Could you check a few things on this drawing? It's one solid part, dimensions in mm from its lowest x, y, z. A direction names the side the tool comes from. Coordinates: 2 decimals unless noted, no trailing zeros. Loops run counter-clockwise (first coordinate to the right, second up) from the corner with the lowest first, then second, coordinate; pieces in that order, holes last. Notation, with made-up numbers: (41.25, 17.5) -> (56.25, 17.5) arc R25 ccw to (56.25, 48.5) -> close; hole circle Ø6 at (-26.5, 41). An arc over 180 degrees is marked (long way). One line per question, with ' | ' between items.
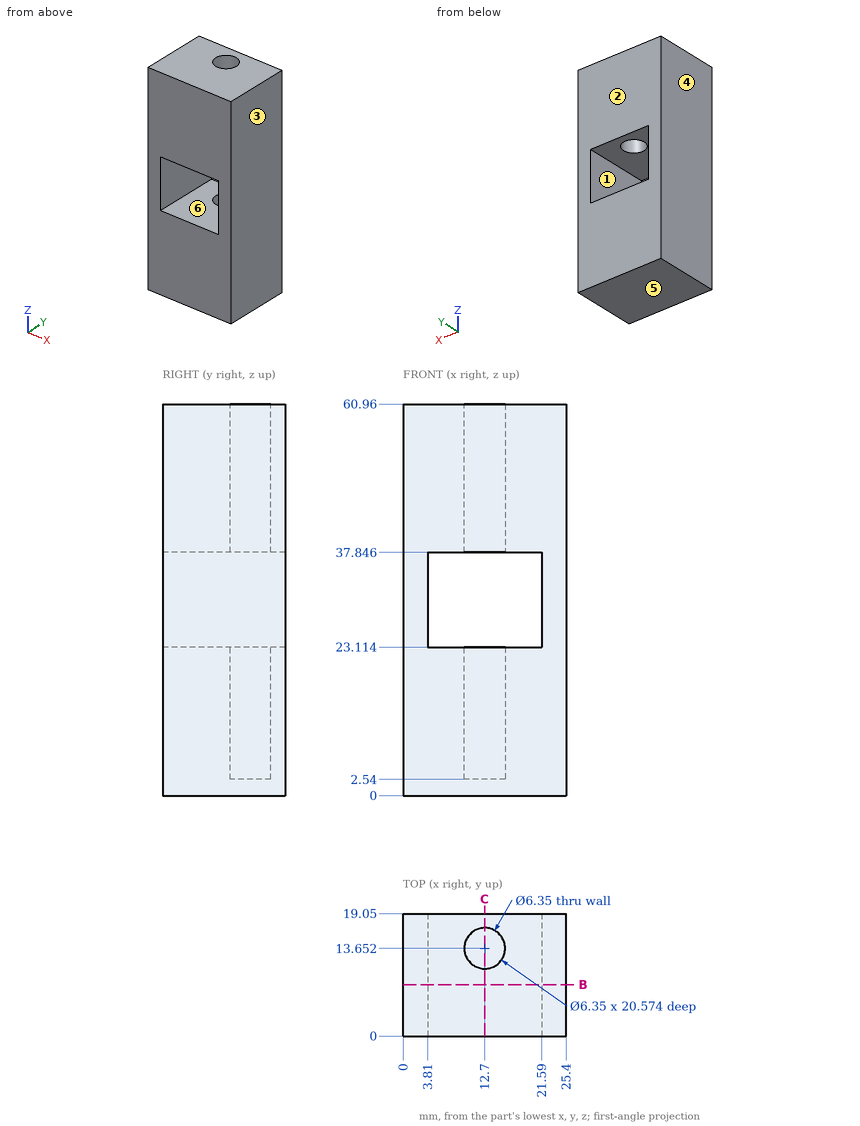
1) If we section it at C-C on x = 12.7: Give the number of separate pieces and of enclosed holes in the cut face, and give its area (3 significant figures).
Data:
separate pieces: 3 | enclosed holes: 0 | area: 603 mm²
2) If we section it at B-B on y = 8: Please give me the cut outline in (x, z) (1 decimal), and give its area (3 significant figures).
Data:
outline: (0, 0) -> (25.4, 0) -> (25.4, 61) -> (0, 61) -> close; hole (3.8, 23.1) -> (21.6, 23.1) -> (21.6, 37.8) -> (3.8, 37.8) -> close | area: 1,290 mm²
3) I need wall thicknesses on line 1 along X through (y, z) = (8.75, 35); line 2 along Z through (x, y) = (5.5, 14.25) (1 decimal); line 3 along Y through (x, z) = (12.7, 48). Which ranges of each line are inside material? Lowest first, please. Write a range as from..to.
Data:
line 1: 0..3.81, 21.59..25.4 | line 2: 0..23.1, 37.8..61 | line 3: 0..10.48, 16.83..19.05
4) On a 3-axis mill with a long thin cutter (end or side, diameter ignored), from which of +Z, -Z, +X, -X, +Y, -Y can I reach the whole of each face in a straight line? I mean the marked faces 5 and 6. Say none if no direction works.
Data:
face 5: -Z, +X, -X, +Y, -Y | face 6: +Y, -Y
5) We'd pull the mould along X, two halves only. Please class the marked faces 1, 2, 3 and 4: pulls with the +X half, pulls with the -X half, needs draft (parallel to the pull), parting line crosses it, or undercut.
Data:
face 1: undercut | face 2: needs draft | face 3: pulls with the +X half | face 4: pulls with the -X half
